Can you work these out from the model? Positions are in its coordinate system, mm. Face numbers are marked on the shaded views. A direction names the side the tool comes from. Give positions to 0.01 mm unless a question says otherwise; leave off trailing zeros. Write each loop counter-clockwise with the first axis right and the second up, starting at its lowest first coordinate (ties: lowest second). Pieces come first, ordered by that corner, then holes. Notation, with made-up numbers: M -32,44.5 L 23,44.5 A21 ccw 23,54.5 Z; hole C -29,40.5 d5. An arc over 180 degrees is marked long. Use CSV: the item, a comma, the result in double quotes. Start each with the question number.
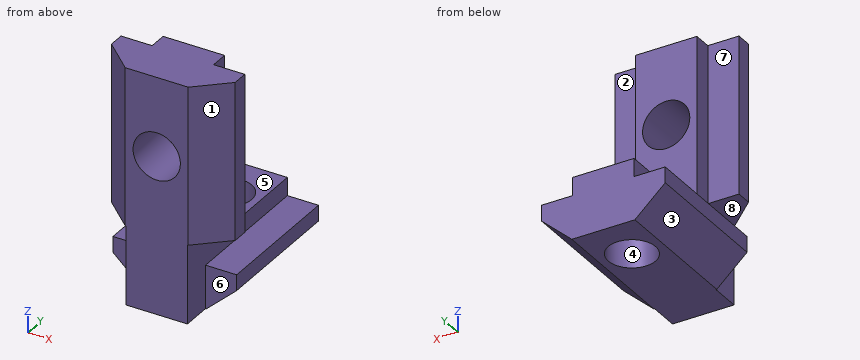
from build123d import *

# Parameters (mm, degrees)
EXTRUDE_1_DEPTH      = 20
EXTRUDE_1_DEPTH_BACK = 0.0001
SKETCH_2_W           = 7.8
SKETCH_2_H           = 7.8
EXTRUDE_2_DEPTH      = 10
EXTRUDE_3_DEPTH      = 13.2
EXTRUDE_3_DEPTH_BACK = 4
SKETCH_4_R           = 3
CUT_EXTRUDE_1_DEPTH  = 11.615262649
SKETCH_5_R           = 3
CUT_EXTRUDE_2_DEPTH  = 8.8
SKETCH_6_W           = 7.8
SKETCH_6_H           = 2.815262649
CUT_EXTRUDE_3_DEPTH  = 21.0001


with BuildPart() as part:
    # Эскиз1 → Бобышка-Вытянуть1 (new body, two sides)
    with BuildSketch(Plane.XY) as extrude_1_sk:
        Polygon((-3.9, 8.315262649), (3.9, 8.315262649), (3.9, 3.2), (7.85, 3.2), (7.85, 1.2), (4, -2.3), (-4, -2.3), (-7.85, 1.2), (-7.85, 3.2), (-3.9, 3.2), align=None)
    extrude(amount=EXTRUDE_1_DEPTH)
    extrude(extrude_1_sk.sketch, amount=-EXTRUDE_1_DEPTH_BACK)

    # Эскиз2 → Бобышка-Вытянуть2 (add)
    with BuildSketch(Plane(origin=(0, 0, -0.0001), x_dir=(-1, 0, 0), z_dir=(0, 0, -1))):
        with Locations((0, 1.6)):
            Rectangle(SKETCH_2_W, SKETCH_2_H)
    extrude(amount=EXTRUDE_2_DEPTH)

    # Эскиз3 → Бобышка-Вытянуть3 (add, two sides)
    with BuildSketch(Plane(origin=(0, 5.5, 0), x_dir=(1, 0, 0), z_dir=(0, 1, 0))) as extrude_3_sk:
        Polygon((3.9, 2.2001), (-3.9, 2.2001), (-3.9, 4.5001), (-7.85, 4.5001), (-7.85, 6.5001), (-4, 10.0001), (4, 10.0001), (7.85, 6.5001), (7.85, 4.5001), (3.9, 4.5001), align=None)
    extrude(amount=EXTRUDE_3_DEPTH)
    extrude(extrude_3_sk.sketch, amount=-EXTRUDE_3_DEPTH_BACK)

    # Эскиз4 → Вырез-Вытянуть1 (cut, through all)
    with BuildSketch(Plane(origin=(0, 8.315262649, 0), x_dir=(1, 0, 0), z_dir=(0, 1, 0))):
        with Locations(Location((0, -10, 0), (0, 0, 180))):  # turned: the seam where the file's is
            Circle(SKETCH_4_R)
    extrude(amount=-CUT_EXTRUDE_1_DEPTH, mode=Mode.SUBTRACT)

    # Эскиз5 → Вырез-Вытянуть2 (cut, through all)
    with BuildSketch(Plane.XY.offset(-2.2001)):
        with Locations((0, 12.7)):
            Circle(SKETCH_5_R)
    extrude(amount=-CUT_EXTRUDE_2_DEPTH, mode=Mode.SUBTRACT)

    # Эскиз6 → Вырез-Вытянуть3 (cut, through all)
    with BuildSketch(Plane(origin=(0, 0, -0.0001), x_dir=(-1, 0, 0), z_dir=(0, 0, -1))):
        with Locations((0, 6.907631325)):
            Rectangle(SKETCH_6_W, SKETCH_6_H)
    extrude(amount=-CUT_EXTRUDE_3_DEPTH, mode=Mode.SUBTRACT)


solid = part.part
(1) Which directions (+Z, -Z, +X, -X, +Y, -Y) give clear straight access to the entire face, cutting with the end or side of a thin tool? Please do the marked faces 5, 6, 7 and 8.
(2) I want a section at A-A (x = 0). Write out the boundary of the cut face in (y, z).
(3) Will these pins go through, and if not, where does the flat tip stop? pin 1 Ø2 at (x, y) = (5.5, -0.5) entering from -Z; pin 2 Ø2 at (x, z) = (-5.5, 11.5) entering from +Y; pin 3 Ø2 at (y, z) = (16, -2) entering from -X.
(4) I want a section at B-B (y = 4.5). Write out the boundary of the cut face in (x, z).
(5) I want a section at D-D (y = 12.7). Write out the boundary of the cut face in (x, z), and give its area (3 significant figures).
(6) Please list where these lines run through material, in increasing order: L1, parallel to Y at x = 0, z = -6.5; L2, parallel to Z at x = 0, y = -0.5; L3, parallel to Y at x = -1.5, z = -1. Write a range as [from, to].
(7) I want a section at C-C (z = 10). Write out the boundary of the cut face in (x, y).
(8) Thinking about a two-plate mould opening in X: for the marked faces 1, 2, 3 and 4, which applies, released by +X, released by -X, zero draft, split by the parting line, or undercut?
Geometry results:
1,face 5,"+Z, +X, -X, +Y"
1,face 6,"-Z, +X, -Y"
1,face 7,"+Z, -X, +Y"
1,face 8,"-X, +Y, -Y"
2,outline,"M -2.3,-10 L 9.7,-10 L 9.7,-2.2 L 5.5,-2.2 L 5.5,7 L -2.3,7 Z; M -2.3,13 L 5.5,13 L 5.5,20 L -2.3,20 Z; M 15.7,-10 L 18.7,-10 L 18.7,-2.2 L 15.7,-2.2 Z"
3,pin 1,"stops at z = 0"
3,pin 2,"stops at y = 3.2"
3,pin 3,"stops at x = -3.9"
4,outline,"M -7.85,-6.5 L -4,-10 L 4,-10 L 7.85,-6.5 L 7.85,-4.5 L 3.9,-4.5 L 3.9,20 L -3.9,20 L -3.9,-4.5 L -7.85,-4.5 Z; hole C 0,10 d6"
5,outline,"M -7.85,-6.5 L -4,-10 L -3,-10 L -3,-2.2 L -3.9,-2.2 L -3.9,-4.5 L -7.85,-4.5 Z; M 3,-10 L 4,-10 L 7.85,-6.5 L 7.85,-4.5 L 3.9,-4.5 L 3.9,-2.2 L 3,-2.2 Z"
5,area,"44.0 mm2"
6,L1,"y = [-2.3, 9.7], [15.7, 18.7]"
6,L2,"z = [-10, 7], [13, 20]"
6,L3,"y = [-2.3, 5.5]"
7,outline,"M -7.85,1.2 L -4,-2.3 L -3,-2.3 L -3,5.5 L -3.9,5.5 L -3.9,3.2 L -7.85,3.2 Z; M 3,-2.3 L 4,-2.3 L 7.85,1.2 L 7.85,3.2 L 3.9,3.2 L 3.9,5.5 L 3,5.5 Z"
8,face 1,"released by +X"
8,face 2,"zero draft"
8,face 3,"released by -X"
8,face 4,"undercut"
